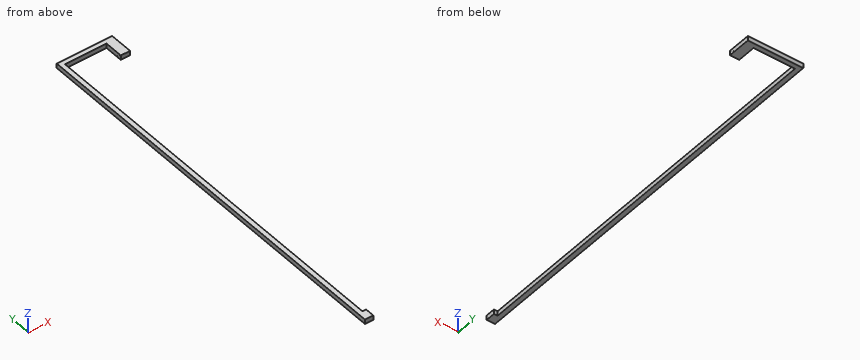
Solid Edge part; units mm, degrees
sketch "Sketch1" plane through (0, 0, 0) normal (0, 0, -1) x (-1, 0, 0)
  line L0 (-110.5657, -295.5663) -> (-110.5657, 1784.4337)
  line L1 (-110.5657, 1784.4337) -> (-335.5657, 1784.4337)
  line L2 (-335.5657, 1784.4337) -> (-335.5657, 1684.4337)
  line L3 (-335.5657, 1684.4337) -> (-385.5657, 1684.4337)
  line L4 (-385.5657, 1684.4337) -> (-385.5657, 1809.4337)
  line L5 (-385.5657, 1809.4337) -> (-85.5657, 1809.4337)
  line L6 (-85.5657, 1809.4337) -> (-85.5657, -345.5663)
  line L7 (-85.5657, -345.5663) -> (-130.5657, -345.5663)
  line L8 (-130.5657, -345.5663) -> (-130.5657, -295.5663)
  line L9 (-130.5657, -295.5663) -> (-110.5657, -295.5663)
extrude "Protrusion1" add sketch "Sketch1" against normal blind 25
hole "Hole_1" at (335.5657, 1688.4337, 21) direction (1, 0, 0) diameter 3.242 end up to next
hole "Hole1" at (335.5657, 1710.4337, 4) direction (1, 0, 0) diameter 3.242 end up to next
chamfer "Chamfer_1" distance 1 angle 45 2 edges at (335.5657, 1688.4337, 22.621) (335.5657, 1710.4337, 5.621)
Check sheet for the modelled part. Datum: model origin and axes. Units: mm. Round coordinates to 2 decimals unless told otherwise and drop trailing zeros. Write each loop counter-clockwise with the first axis right and the second up, starting at its lowest first coordinate (ties: lowest second). Pieces come first, ordered by that corner, then holes. Notation, with made-up numbers: (-15.75, -37.75) - (27.25, -37.75) arc R33 ccw to (27.25, -5.75) - close; hole circle Ø6 at (-9.75, 67). An arc over 180 degrees is marked (long way). Return JSON: item names as keys, results as strings.
Q1. Depth check by flat-ended pin: P1, Ø7.5, axis at x = 187, z = 8.5, coming from the -Y side; P2, Ø12.5, axis at x = 362, z = 14.5, coming from the -Y side; P3, Ø1.5, axis at y = 689.5, z = 21, coming from the +X side. Enter the tip coordinate at first touch or a pass-through.
Returned:
{"P1": "stops at y = 1784.43", "P2": "stops at y = 1684.43", "P3": "stops at x = 110.57"}
Q2. Cross-section at A-A (z = 13). Record the boundary of the cut face in (x, y), then the cut area to 4 significant figures.
Returned:
{"outline": "(85.57, -345.57) - (130.57, -345.57) - (130.57, -295.57) - (110.57, -295.57) - (110.57, 1784.43) - (335.57, 1784.43) - (335.57, 1684.43) - (385.57, 1684.43) - (385.57, 1809.43) - (85.57, 1809.43) - close", "area": "66,750 mm²"}
Q3. Cross-section at C-C (y = 66.5). Record the boundary of the cut face in (x, z).
Returned:
{"outline": "(85.57, 0) - (110.57, 0) - (110.57, 25) - (85.57, 25) - close"}
Q4. Scan lines: L1, parallel to Y at x = 365, z = 21; L2, parallel to Y at x = 353, z = 4; L3, parallel to X at y = 1220.5, z = 6.25. Record each from-to range of solid material in increasing order. Write a range as from..to.
Returned:
{"L1": "y = 1684.43..1686.81, 1690.05..1809.43", "L2": "y = 1684.43..1708.81, 1712.05..1809.43", "L3": "x = 85.57..110.57"}
Q5. Cross-section at B-B (x = 265.5). Record the boundary of the cut face in (y, z), then the cut area to 3 significant figures.
Returned:
{"outline": "(1784.43, 0) - (1809.43, 0) - (1809.43, 25) - (1784.43, 25) - close", "area": "625 mm²"}
